The listing builds one solid part. Answer for the finished solid, in the listing's coordinates (mm). A direction names the side the tool comes from. Coordinates: 2 decimals unless noted, no trailing zeros. Order: outer loops, then holes, each group sorted by start corner. A loop starts at its lowest first (then second) coordinate and runs counter-clockwise, first axis right, second up. Notation, with made-up numbers: (68.5, -18.75) - (97.5, -18.75) arc R31 ccw to (97.5, 16.25) - close; hole circle Ø3 at (64, -6.75). An arc over 180 degrees is marked (long way). One line per item, written item: value. Start each with the question number.
```python
from build123d import *

# Parameters (mm, degrees)
BOSS_EXTRUDE1_DEPTH = 6
SKETCH2_W           = 34
SKETCH2_H           = 99
CUT_EXTRUDE1_DEPTH  = 4
SKETCH4_R           = 1.9
CUT_EXTRUDE2_DEPTH  = 7
SKETCH5_R           = 1.8
SKETCH5_R_2         = 1.25
CUT_EXTRUDE3_DEPTH  = 10
SKETCH6_R           = 1.25
CUT_EXTRUDE4_DEPTH  = 10
SKETCH7_R           = 1.25
CUT_EXTRUDE5_DEPTH  = 10
SKETCH8_R           = 1.8
SKETCH8_R_2         = 1.25
BOSS_EXTRUDE2_DEPTH = 6


with BuildPart() as part:
    # Sketch1 → Boss-Extrude1 (new body)
    with BuildSketch(Plane(origin=(0, 0, 0), x_dir=(1, 0, 0), z_dir=(0, 1, 0))):
        Polygon((-41.317279836, -84.379169784), (-41.317279836, -89.379169784), (41.317279836, -89.379169784), (41.317279836, -84.379169784), (81.317279836, -15.097137481), (0, 66.220142355), (-81.317279836, -15.097137481), align=None)
    extrude(amount=BOSS_EXTRUDE1_DEPTH)

    # Sketch2 → Cut-Extrude1 (cut)
    with BuildSketch(Plane(origin=(0, 6, 0), x_dir=(1, 0, 0), z_dir=(0, 1, 0))):
        with Locations((0.002279836, -39.879169784)):
            Rectangle(SKETCH2_W, SKETCH2_H)
    extrude(amount=-CUT_EXTRUDE1_DEPTH, mode=Mode.SUBTRACT)

    # Sketch4 → Cut-Extrude2 (cut, through all)
    with BuildSketch(Plane(origin=(0, 6, 0), x_dir=(1, 0, 0), z_dir=(0, 1, 0))):
        with Locations((-22.627416998, 25.207949047)):
            Circle(SKETCH4_R)
        with Locations((-40.305086528, 7.530279517)):
            Circle(SKETCH4_R)
        with Locations((-55.979629628, -32.983234986)):
            Circle(SKETCH4_R)
        with Locations((-43.479629628, -54.633870081)):
            Circle(SKETCH4_R)
        with Locations((43.479629628, -54.633870081)):
            Circle(SKETCH4_R)
        with Locations((55.979629628, -32.983234986)):
            Circle(SKETCH4_R)
        with Locations((22.627416998, 25.207949047)):
            Circle(SKETCH4_R)
        with Locations((40.305086528, 7.530279517)):
            Circle(SKETCH4_R)
    extrude(amount=-CUT_EXTRUDE2_DEPTH, mode=Mode.SUBTRACT)

    # Sketch5 → Cut-Extrude3 (cut)
    with BuildSketch(Plane(origin=(0, 6, 0), x_dir=(1, 0, 0), z_dir=(0, 1, 0))):
        with Locations((-28.497720164, -73.379169784)):
            Circle(SKETCH5_R)
        with Locations((28.502279836, -73.379169784)):
            Circle(SKETCH5_R)
        with Locations((26.002279836, -86.379169784)):
            Circle(SKETCH5_R_2)
        with Locations((-25.997720164, -86.379169784)):
            Circle(SKETCH5_R_2)
    extrude(amount=-CUT_EXTRUDE3_DEPTH, mode=Mode.SUBTRACT)

    # Sketch6 → Cut-Extrude4 (cut)
    with BuildSketch(Plane(origin=(0, 2, 0), x_dir=(1, 0, 0), z_dir=(0, 1, 0))):
        with Locations((7.002279836, 2.120830216)):
            Circle(SKETCH6_R)
        with Locations((-6.997720164, 2.120830216)):
            Circle(SKETCH6_R)
        with Locations((-6.997720164, -66.879169784)):
            Circle(SKETCH6_R)
        with Locations((7.002279836, -66.879169784)):
            Circle(SKETCH6_R)
    extrude(amount=-CUT_EXTRUDE4_DEPTH, mode=Mode.SUBTRACT)

    # Sketch7 → Cut-Extrude5 (cut)
    with BuildSketch(Plane(origin=(0, 6, 0), x_dir=(1, 0, 0), z_dir=(0, 1, 0))):
        with Locations((-32.497720164, -73.379169784)):
            Circle(SKETCH7_R)
        with Locations((-24.497720164, -73.379169784)):
            Circle(SKETCH7_R)
    cut_extrude5 = extrude(amount=-CUT_EXTRUDE5_DEPTH, mode=Mode.SUBTRACT)

    # Mirror1: Cut-Extrude5 across plane
    add(cut_extrude5.mirror(Plane(origin=(0, 0, 0), x_dir=(0, 0, 1), z_dir=(1, 0, 0))), mode=Mode.SUBTRACT)

    # Sketch8 → Boss-Extrude2 (add)
    with BuildSketch(Plane(origin=(0, 6, 0), x_dir=(1, 0, 0), z_dir=(0, 1, 0))):
        with Locations((-28.497720164, -73.379169784)):
            Circle(SKETCH8_R)
        with Locations((-25.997720164, -86.379169784)):
            Circle(SKETCH8_R_2)
    boss_extrude2 = extrude(amount=-BOSS_EXTRUDE2_DEPTH)

    # Mirror2: Boss-Extrude2 across plane
    add(boss_extrude2.mirror(Plane(origin=(0, 0, 0), x_dir=(0, 0, 1), z_dir=(1, 0, 0))))


solid = part.part
```
(1) Consider probe 1 along Z at (x, y) = (42, 3.5); probe 2 along X at (y, z) = (3.55, -45.5); probe 3 along Y at (x, z) = (9.5, 6). Determine where each line is inside the solid, lowest interval first.
(2) For faces 1 (the face through (17.002, 4, 41)), 2 (the face through (-44.88, 3.04, 53.35)), 3 (the face through (-41.317, 3, 87)), determine the directions among +Z, -Z, +X, -X, +Y, -Y from which every point of the face is accessible in a straight line to the end or side of a thin tool.
(3) Flat-ended cylindrical pins translate along their axes: pin 1 Ø2.5 at (y, z) = (2.5, 87.5) entering from -X; pin 2 Ø3 at (x, y) = (30.5, 4) entering from -Z; pin 3 Ø2 at (y, z) = (5, 20.5) entering from -X; pin 4 Ø3.5 at (x, z) = (40.31, -7.53) entering from -Y. Find the tip coordinate at first contact, or state that the pin passes through.
(4) For a pull along Y with two mould halves and no side action, classify faces 4 (the face through (1, 0, 28)), 5 (the face through (-20.815, 3.042, -25.779)) as pulls with the +Y half, pulls with the -Y half, needs draft (parallel to the pull), parting line crosses it, or undercut.
(5) The part is cut by section C-C on z = 77.5. Determine the outline of the cut face in (x, y), plus the area to 3 significant figures.
(6) The part is cut by section A-A on z = 13. Determine the outline of the cut face in (x, y), plus the area to 3 significant figures.
(7) The part is cut by section D-D on x = -67.5. Determine the outline of the cut face in (y, z).
(8) The part is cut by section B-B on x = 70. Determine the outline of the cut face in (y, z), plus the area to 3 significant figures.
Completed:
1. probe 1: z = -24.22 to -8.39, -6.67 to 53.44, 55.83 to 83.2
1. probe 2: x = -20.72 to 20.72
1. probe 3: y = 0 to 2
2. face 1: +Z, +Y
2. face 2: +Y, -Y
2. face 3: +Z, -X, +Y, -Y
3. pin 1: stops at x = -41.32
3. pin 2: stops at z = -37.22
3. pin 3: stops at x = -78.78
3. pin 4: passes through
4. face 4: pulls with the -Y half
4. face 5: needs draft
5. outline: (-45.29, 0) - (45.29, 0) - (45.29, 6) - (17, 6) - (17, 2) - (-17, 2) - (-17, 6) - (-45.29, 6) - close
5. area: 407 mm2
6. outline: (-79.22, 0) - (79.22, 0) - (79.22, 6) - (17, 6) - (17, 2) - (-17, 2) - (-17, 6) - (-79.22, 6) - close
6. area: 815 mm2
7. outline: (0, 1.28) - (6, 1.28) - (6, 39.03) - (0, 39.03) - close
8. outline: (0, 3.78) - (6, 3.78) - (6, 34.7) - (0, 34.7) - close
8. area: 186 mm2
